```python
from build123d import *

# Parameters (mm, degrees)
F2_R     = 27.048464
F3_DEPTH = 76.2
F4_R     = 10.765067
F5_DEPTH = 76.2
F6_R     = 5.378354
F7_DEPTH = 76.2


with BuildPart() as f1:
    # F0 (on Front) → F1 (revolve)
    with BuildSketch(Plane.XZ):
        Polygon((8.565648, -9.424497), (-67.634352, -9.424497), (-67.634352, -60.224497), (-16.834352, -60.224497), (-16.834352, -34.824497), (33.965648, -34.824497), (33.965648, -60.224497), (59.365648, -60.224497), (59.365648, 66.775503), (8.565648, 66.775503), align=None)
    revolve(axis=Axis((59.365648, 0, 3.275503), (0, 0, 1)))

    # F2 (on face) → F3 (join)
    with BuildSketch(Plane.XY.offset(66.775503)):
        with Locations((59.365648, 0)):
            Circle(F2_R)
    extrude(amount=F3_DEPTH)

    # F4 (on face) → F5 (join)
    with BuildSketch(Plane.XY.offset(142.975503)):
        with Locations((59.365648, 0)):
            Circle(F4_R)
    extrude(amount=F5_DEPTH)

    # F6 (on face) → F7 (join)
    with BuildSketch(Plane.XY.offset(219.175503)):
        with Locations((59.365648, 0)):
            Circle(F6_R)
    extrude(amount=F7_DEPTH)


solid = f1.part
```
Check sheet for the modelled part. Datum: model origin and axes. Units: mm. A direction names the side the tool comes from. Give positions to 0.01 mm unless a question says otherwise; leave off trailing zeros. Write each loop counter-clockwise with the first axis right and the second up, starting at its lowest first coordinate (ties: lowest second). Pieces come first, ordered by that corner, then holes. Notation, with made-up numbers: (75.25, -30.5) - (94.25, -30.5) arc R38 ccw to (94.25, 8.5) - close; hole circle Ø4 at (30.25, 89). An arc over 180 degrees is marked (long way). Answer as a JSON object with one key per item and string values. Group by question number.
1) Sectioned sample at D-D (z = 259.5). Record the cut outline in (x, y), then the cut area to 3 significant figures.
2) Release check for a two-part mould opening along X. For faces 4 (the face through (27, -1, -34.824)), 5 (the face through (10.91, -15.26, 28.14)), 6 (the face through (59, -12, 142.976)) record: pulls with the +X half, pulls with the -X half, needs draft (parallel to the pull), parting line crosses it, or undercut.
3) Access from +Z, -Z, +X, -X, +Y, -Y to the whole of each face (thin tool, end or side, straight path). Record for faces 1 (the face through (-13.316, -22.888, -47.347)), 2 (the face through (5, 55, -60.224)), 3 (the face through (64.334, -2.06, 256.742)).
4) Thickness scan on probe 1 along X at (y, z) = (0, -48); probe 2 along Z at (x, y) = (160.5, 39); probe 3 along Z at (x, y) = (63.5, 69.5). Record the ranges inside material, lowest first. Write a range as from..to.
5) Sectioned sample at A-A (y = 0). Record the cut outline in (x, z), then the cut area to 3 significant figures.
6) Sectioned sample at C-C (z = 8). Record the cut outline in (x, y), then the cut area to 3 significant figures.
7) Sectioned sample at B-B (x = 79). Record the cut outline in (y, z).
8) Depth check by flat-ended pin: P1, Ø8, axis at x = 28.5, y = -67.5, coming from the -Z side; P2, Ø2, axis at x = 25, y = -59, coming from the +Z side; P3, Ø5, axis at y = 22, z = 133, coming from the +X side. Enter the tip coordinate at first touch or a pass-through.
Geometry results:
{
 "1": {"outline": "circle Ø10.76 at (59.37, 0)", "area": "90.9 mm^2"},
 "2": {"face 4": "undercut", "face 5": "parting line crosses it", "face 6": "needs draft"},
 "3": {"face 1": "-Z", "face 2": "-Z, +X, -X, +Y, -Y", "face 3": "+Z"},
 "4": {"probe 1": "x = -67.63..-16.83, 33.97..84.77, 135.57..186.37", "probe 2": "z = -60.22..-9.42", "probe 3": "z = -34.82..-9.42"},
 "5": {"outline": "(-67.63, -60.22) - (-16.83, -60.22) - (-16.83, -34.82) - (33.97, -34.82) - (33.97, -60.22) - (84.77, -60.22) - (84.77, -34.82) - (135.57, -34.82) - (135.57, -60.22) - (186.37, -60.22) - (186.37, -9.42) - (110.17, -9.42) - (110.17, 66.78) - (86.41, 66.78) - (86.41, 142.98) - (70.13, 142.98) - (70.13, 219.18) - (64.74, 219.18) - (64.74, 295.38) - (53.99, 295.38) - (53.99, 219.18) - (48.6, 219.18) - (48.6, 142.98) - (32.32, 142.98) - (32.32, 66.78) - (8.57, 66.78) - (8.57, -9.42) - (-67.63, -9.42) - close", "area": "24,600 mm^2"},
 "6": {"outline": "circle Ø101.6 at (59.37, 0)", "area": "8,110 mm^2"},
 "7": {"outline": "(-125.47, -60.22) - (-73.63, -60.22) - (-73.63, -34.82) - (-16.11, -34.82) - (-16.11, -60.22) - (16.11, -60.22) - (16.11, -34.82) - (73.63, -34.82) - (73.63, -60.22) - (125.47, -60.22) - (125.47, -9.42) - (46.85, -9.42) - (46.85, 66.78) - (18.6, 66.78) - (18.6, 142.98) - (-18.6, 142.98) - (-18.6, 66.78) - (-46.85, 66.78) - (-46.85, -9.42) - (-125.47, -9.42) - close"},
 "8": {"P1": "stops at z = -60.22", "P2": "stops at z = -9.42", "P3": "stops at x = 78.11"}
}
